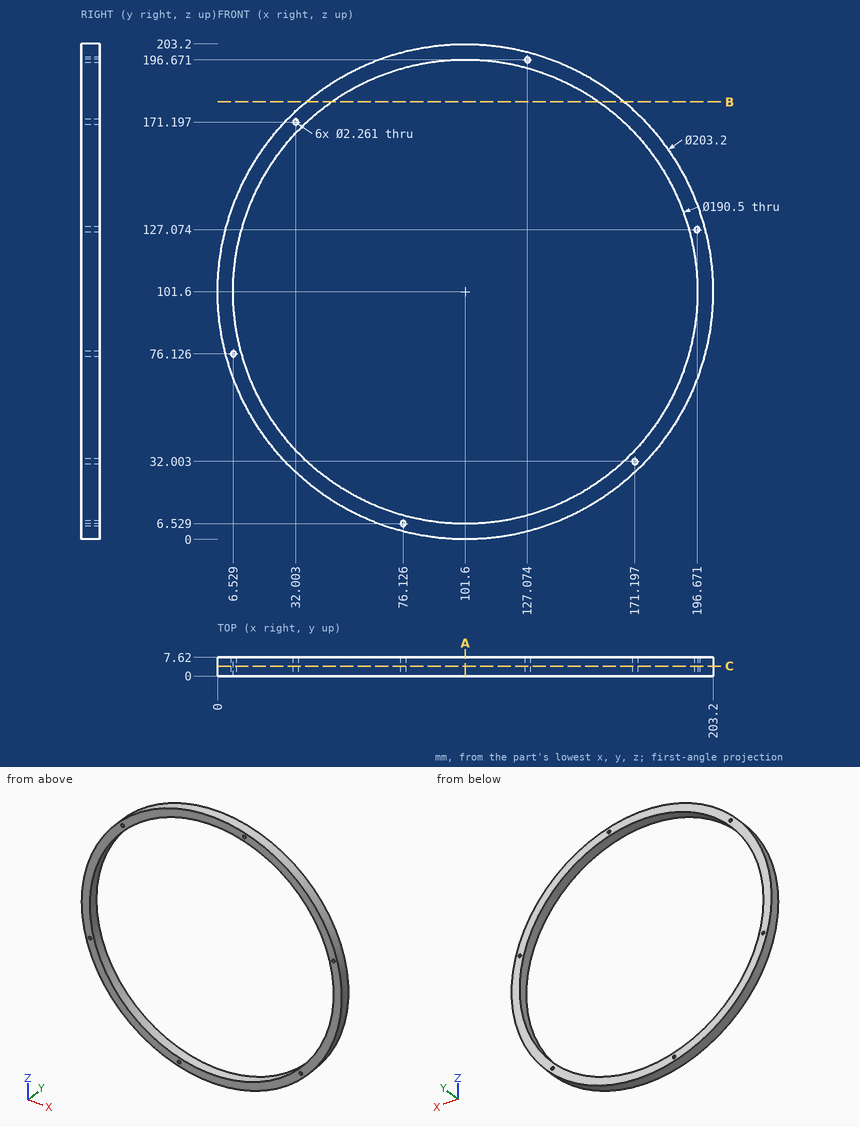
Answer from the drawing. Dimensions are ordinates in mm from the lowest x, y and z of the part. Coordinates: 2 decimals unless noted, no trailing zeros. Loops run counter-clockwise (first coordinate to the right, second up) from the corner with the lowest first, then second, coordinate; pieces in that order, holes last. Notation, with made-up numbers: (61.5, -13.5) -> (78.5, -13.5) arc R13 cw to (78.5, 2.5) -> close; hole circle Ø3 at (83, -29). An arc over 180 degrees is marked (long way). Return JSON: item names as keys, results as strings.
Item 1: Find the intervals of material crossed by probe 1 along X at (y, z) = (1.75, 102); probe 2 along X at (y, z) = (1, 170.5) (1 decimal); probe 3 along Z at (x, y) = (63, 1), in increasing order.
Answers:
{"probe 1": "x = 0 to 6.35, 196.85 to 203.2", "probe 2": "x = 26.9 to 31.1, 32.9 to 35.8, 167.4 to 176.3", "probe 3": "z = 7.62 to 14.52, 188.68 to 195.58"}
Item 2: Find section B-B (z = 179.5). Determine the outline of the cut face in (x, y).
Answers:
{"outline": "(36.38, 0) -> (46.79, 0) -> (46.79, 7.62) -> (36.38, 7.62) -> close; (156.41, 0) -> (166.82, 0) -> (166.82, 7.62) -> (156.41, 7.62) -> close"}
Item 3: Find section A-A (x = 101.6). Determine the outline of the cut face in (y, z).
Answers:
{"outline": "(0, 0) -> (7.62, 0) -> (7.62, 6.35) -> (0, 6.35) -> close; (0, 196.85) -> (7.62, 196.85) -> (7.62, 203.2) -> (0, 203.2) -> close"}
Item 4: Find section C-C (y = 4). Count the separate pieces of the cut face and the enclosed holes in it, plus the area to 3 significant figures.
Answers:
{"separate pieces": "1", "enclosed holes": "7", "area": "3,900 mm2"}
Item 5: Flat-ended cylindrical pins translate along their axes: P1, Ø3, axis at y = 6, z = 88.5, coming from the +X side; P2, Ø3, axis at y = 2, z = 149.5, coming from the -X side (1 decimal); P3, Ø2, axis at x = 110, y = 5, coming from the +Z side. Find the tip coordinate at first contact, or state that the pin passes through.
Answers:
{"P1": "stops at x = 202.54", "P2": "stops at x = 11.2", "P3": "stops at z = 202.93"}
